Could you check a few things on this drawing? It's one solid part, dimensions in mm from its lowest x, y, z. Give positions to 0.01 mm unless a question says otherwise; leave off trailing zeros. Order: outer loops, then holes, each group sorted by start corner. A loop starts at its lowest first (then second) coordinate and runs counter-clockwise, first axis right, second up.
(1) If I drill on probe 1 along X at (y, z) = (2.75, 26.5); probe 2 along Z at (x, y) = (24, 1); probe 3 along X at (y, z) = (3.5, 22), over which ranges is the centre line in solid material (lowest first)?
(2) Imagine slicing it at C-C, the plane z = 40. Write out the boundary of the cut face in (x, y), then the cut area to 3 significant figures.
(3) Imagine slicing it at A-A, the plane z = 14.5. Write out the boundary of the cut face in (x, y).
(4) Imagine slicing it at B-B, the plane y = 9. Write out the boundary of the cut face in (x, z) (3 decimals).
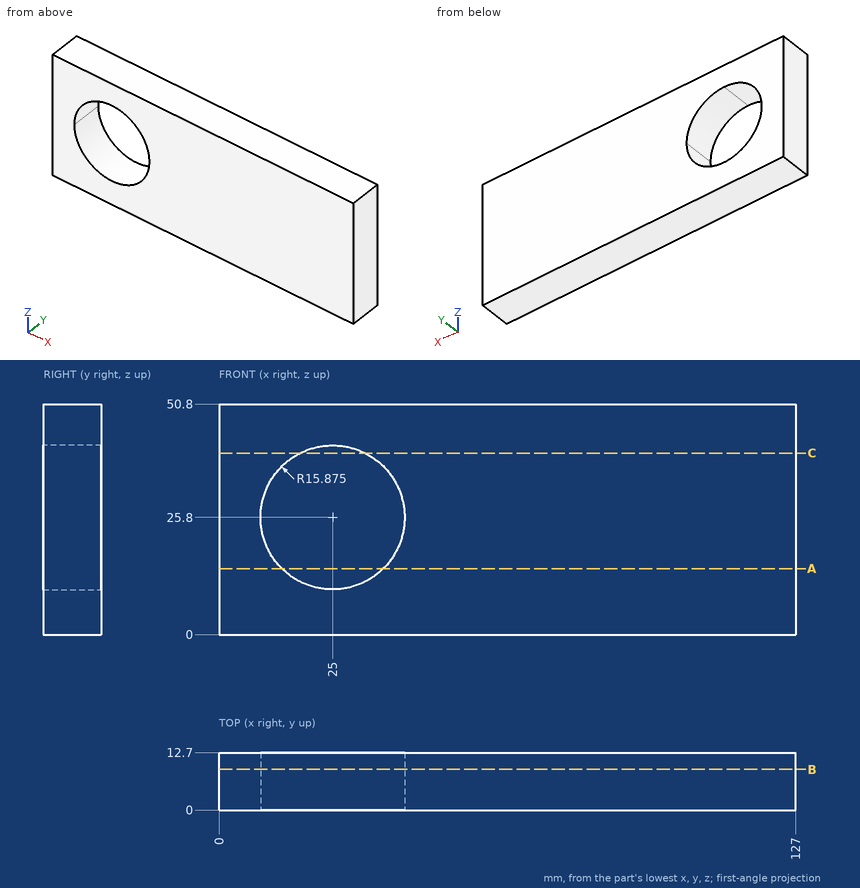
Answer block:
1. probe 1: x = 0 to 9.14, 40.86 to 127
1. probe 2: z = 0 to 9.96, 41.64 to 50.8
1. probe 3: x = 0 to 9.59, 40.41 to 127
2. outline: (0, 0) - (17.9, 0) - (17.9, 12.7) - (0, 12.7) - close; (32.1, 0) - (127, 0) - (127, 12.7) - (32.1, 12.7) - close
2. area: 1,430 mm2
3. outline: (0, 0) - (13.85, 0) - (13.85, 12.7) - (0, 12.7) - close; (36.15, 0) - (127, 0) - (127, 12.7) - (36.15, 12.7) - close
4. outline: (0, 0) - (127, 0) - (127, 50.8) - (0, 50.8) - close; hole circle Ø31.75 at (25, 25.8)
